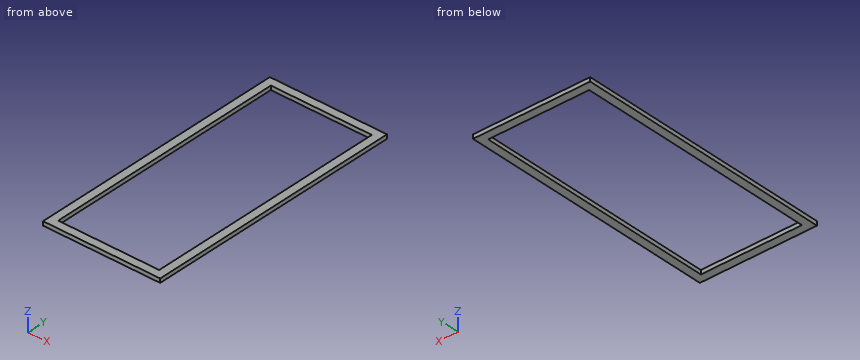
from build123d import *

# Parameters (mm, degrees)
SKETCH2_W           = 29
SKETCH2_H           = 64
BOSS_EXTRUDE1_DEPTH = 1
SKETCH3_W           = 25
SKETCH3_H           = 60
CUT_EXTRUDE4_DEPTH  = 1


with BuildPart() as part:
    # Sketch2 → Boss-Extrude1 (new body)
    with BuildSketch(Plane.XY):
        Rectangle(SKETCH2_W, SKETCH2_H)
    extrude(amount=-BOSS_EXTRUDE1_DEPTH)

    # Sketch3 → Cut-Extrude4 (cut)
    with BuildSketch(Plane.XY):
        Rectangle(SKETCH3_W, SKETCH3_H)
    extrude(amount=-CUT_EXTRUDE4_DEPTH, mode=Mode.SUBTRACT)


solid = part.part
Design review of the part built by this model. Coordinates are the model's own, in mm. Round coordinates to 2 decimals unless told otherwise and drop trailing zeros. Write each loop counter-clockwise with the first axis right and the second up, starting at its lowest first coordinate (ties: lowest second). Pieces come first, ordered by that corner, then holes. Notation, with made-up numbers: M 6,65 L 14,65 A24 cw 14,97 Z; hole C -19.5,-6.75 d4. An arc over 180 degrees is marked long. One line per item, written item: value. Start each with the question number.
1. To check wall thickness, follow probe 1 along Y at (x, z) = (-10, -0.25); probe 2 along X at (y, z) = (17, -0.55). State the ranges of each line that lie inside material, in increasing order. Write a range as from..to.
2. Take a section at B-B on x = 11. State the section outline as (y, z) points, then the cut area to 3 significant figures.
3. Take a section at A-A on y = -23. State the section outline as (x, z) points.
4. Take a section at C-C on z = -0.8. State the section outline as (x, y) points, then the cut area to 3 significant figures.
Computed:
1. probe 1: y = -32..-30, 30..32
1. probe 2: x = -14.5..-12.5, 12.5..14.5
2. outline: M -32,-1 L -30,-1 L -30,0 L -32,0 Z; M 30,-1 L 32,-1 L 32,0 L 30,0 Z
2. area: 4.00 mm²
3. outline: M -14.5,-1 L -12.5,-1 L -12.5,0 L -14.5,0 Z; M 12.5,-1 L 14.5,-1 L 14.5,0 L 12.5,0 Z
4. outline: M -14.5,-32 L 14.5,-32 L 14.5,32 L -14.5,32 Z; hole M -12.5,-30 L 12.5,-30 L 12.5,30 L -12.5,30 Z
4. area: 356 mm²
